Work out the finished part from the listing and answer in its coordinate system (mm). A direction names the side the tool comes from. Coordinates: 2 decimals unless noted, no trailing zeros. Order: outer loops, then holes, each group sorted by start corner. A loop starts at its lowest first (then second) coordinate and runs counter-clockwise, first axis right, second up. Notation, with made-up numbers: (-22, -20.75) -> (26, -20.75) arc R19 cw to (26, 5.25) -> close; hole circle Ø7 at (85.5, -20). An arc over 180 degrees is marked (long way). Write item = value, one per line. Start each with the question number.
Q1. Which of the six approach directions +Z, -Z, +X, -X, +Y, -Y give full straight-line access (tool end or side, diameter ignored) to faces 4 (the cylindrical face through (-2.13, -1.03, 4.65)), 5 (the flat face through (-4, -0.952, 0))?
Q2. Straight lines are drawn through the part: L1, parallel to X at y = -1, z = 3.75; L2, parallel to Y at x = 27.5, z = -2.5; L3, parallel to Y at x = 10, z = 0.75. For each, find the intervals that lie inside material, in ascending order. Write a range as from..to.
Q3. Flat-ended cylindrical pins translate along their axes: pin 1 (5 mm diameter, centred on x = 25, z = 2.5, fed in from -Y) (3 decimals); pin 2 (2 mm diameter, centred on x = 18.5, y = 0.5, fed in from +Z) (3 decimals); pin 3 (1.9 mm diameter, centred on x = -4, z = 0.5, fed in from -Y); pin 4 (4 mm diameter, centred on x = 36, y = -2.5, fed in from +Z). Find the tip coordinate at first contact, or state that the pin passes through.
Q4. The part is cut by section A-A, the plane x = 27.5. Determine the outline of the cut face in (y, z) (3 decimals), plus the area to 3 significant figures.
Q5. For a pull along Y with two mould halves and no side action, classify faces 1 (the flat face through (-3.023, 0, 0)), 2 (the cylindrical face through (21.58, -0.69, 3.1)), 3 (the flat face through (0, -2, 4)) as +Y half, -Y half, draft (parallel to the pull), parting line (faces both ways), or undercut.
Autodesk Inventor part; units mm, degrees
ref_plane "IDS_WORKPLANE{1}" through (-5.4864, 0, 0) normal (1, 0, 0) x (0, 0, -1)
ref_plane "Work Plane2" through (41.275, 0, 0) normal (0, 0, -1) x (1, 0, 0)
ref_plane "YZ Plane" through (0, 0, 0) normal (1, 0, 0) x (0, 1, 0)
sketch "Sketch1" plane through (0, 0, 0) normal (0, 0, 1) x (1, 0, 0)
  line L0 (-5.4864, 0) -> (44.45, 0)
  line L1 (44.45, 0) -> (44.45, 3.175)
  line L2 (44.45, 3.175) -> (25.4, 3.175)
  line L3 (25.4, 3.175) -> (24.638, 3.175)
  line L4 (24.638, 3.175) -> (0, 3.175)
  line L5 (0, 3.175) -> (0, 4.7625)
  line L6 (-15.8499, 0) -> (54.5, 0)
  line L7 (0, -0.9693) -> (0, 5.8158)
  line L8 (0, 4.7625) -> (-4.2103, 4.7625)
  arc A0 (-4.2103, 4.7625) -> (-5.4864, 0) centre (4.0386, 0) ccw
  line L9 (25.4, 3.175) -> (0, 3.175) construction
  dimension "d0" = 44.45
  dimension "d1" = 19.05
  dimension "d2" = 0.762
  dimension "d3" = 5.4864
  dimension "d4" = 6.35
  dimension "d5" = 6.35
  dimension "d9" = 9.525
  dimension "d10" = 0
  dimension "d13" = 9.525
revolve "Body" add sketch "Sketch1" angle 360 about axis through (-5.4864, 0, 0) along (1, 0, 0)
ref_plane "IDS_WORKPLANE{1}" through (-5.4864, 0, 0) normal (1, 0, 0) x (0, 0, -1)
sketch "Sketch2" plane through (-5.4864, 0, 0) normal (1, 0, 0) x (0, 0, -1)
  circle A0 centre (0, 0) radius 4.7625
  line L0 (0, -6.6675) -> (0, 6.6675)
  line L1 (6.6675, 0) -> (-6.6675, 0)
  line L2 (-4.7625, 0.9525) -> (4.7625, 0.9525)
  line L3 (4.7625, 0.9525) -> (4.7625, -0.9525)
  line L4 (4.7625, -0.9525) -> (-4.7625, -0.9525)
  line L5 (-4.7625, -0.9525) -> (-4.7625, 0.9525)
  line L6 (-4.7625, 0) -> (4.7625, 0) construction
  line L7 (0, 0.9525) -> (0, -0.9525) construction
  dimension "d15" = 1.905
extrude "Slot" cut sketch "Sketch2" along normal blind 2.4638 contours L1 L0 L2 A0 | L3 L4 A0 | A0 L4 L0 L1 | A0 L2 L3 | L1 A0 L2 L0 | L0 L4 A0 L1 | L5 L2 A0 | A0 L4 L5
thread "Thread"
sketch "Sketch3" plane through (0, 0, 0) normal (0, 0, 1) x (1, 0, 0)
  line L0 (44.45, 0) -> (44.45, 3.175)
  line L1 (44.45, 3.175) -> (25.4, 3.175)
  line L2 (-5.4864, 0) -> (44.45, 0)
  arc A0 (44.45, 0) -> (43.5993, 3.175) centre (38.1, 0) ccw
  line L3 (44.45, -3.175) -> (44.45, 3.175)
  line L4 (43.5993, 3.175) -> (43.5993, 0)
  line L5 (43.5993, 0) -> (44.45, 0)
  dimension "d40" = 6.35
revolve "Fillet1" cut sketch "Sketch3" angle 360 about axis through (-5.4864, 0, 0) along (1, 0, 0) contours A0 L1 L0
chamfer "Chamfer" distance 0.635 angle 45 1 edges at (43.5993, -3.175, 0)
ref_plane "Work Plane2" through (41.275, 0, 0) normal (0, 0, -1) x (1, 0, 0)
fillet "Fillet4" radius 0.7874 1 edges at (0, -3.175, 0)
equation "\"d0\" = NLG"
equation "\"d1\" = GEL"
equation "\"d2\" = GAL"
equation "\"d3\" = KOH"
equation "\"d4\" = GD"
equation "\"d5\" = BDM"
equation "\"d9\" = KOD"
equation "\"d13\" = KR"
equation "\"d15\" = SBR"
equation "\"d16\" = STI"
equation "\"d40\" = GD"
equation "\"d46\" = R"
equation "\"d11\" = GEL"
equation "\"d43\" = 0.5 * RR"
equation "\"GD\" = NND"
equation "\"NLG\" = 44.45"
equation "\"GEL\" = 19.05"
equation "\"KOD\" = 9.525"
equation "\"KOH\" = 5.4864"
equation "\"GAL\" = 0.762"
equation "\"BDM\" = NND"
equation "\"SBR\" = 1.905"
equation "\"STI\" = 2.4638"
equation "\"KEWI\" = 0"
equation "\"KR\" = KOD"
equation "\"d14\" = -KOH"
equation "\"R\" = 0.7874"
equation "\"THREADDIA\" = 6.35"
equation "\"TOA\" = 30deg"
equation "\"KOH1\" = 4.3688"
equation "\"NND\" = 6.35"
equation "\"GD1\" = 4.8387"
equation "\"THREADDESC\" = 1.2345"
properties part number "ANSI B18.6.2 - 1/4-20 UNC - 1.75, SFHCSI" material "Steel, Mild"
Model answer:
q1.face_4 = +X, -X
q1.face_5 = +Z, -Z, -X
q2.L1 = -4.66..0
q2.L2 = -1.96..1.96
q2.L3 = -3.09..3.09
q3.pin_1 = -3.175
q3.pin_2 = 3.175
q3.pin_3 = -4.76
q3.pin_4 = 3.14
q4.outline = circle Ø6.35 at (0, 0)
q4.area = 31.7 mm2
q5.face_1 = undercut
q5.face_2 = parting line
q5.face_3 = draft
